```python
from build123d import *

# Parameters (mm, degrees)
F0_W     = 114.378564
F0_H     = 67.637316
F1_DEPTH = 60.96
F3_DEPTH = 12.7
F5_DEPTH = 12.7
F7_DEPTH = 86.361
F8_R     = 4.717852
F9_DEPTH = 67.638317


with BuildPart() as f1:
    # F0 (on Front) → F1 (new body)
    with BuildSketch(Plane.XZ):
        Rectangle(F0_W, F0_H)
    extrude(amount=-F1_DEPTH)

    # F2 (on face) → F3 (join)
    with BuildSketch(Plane(origin=(0, 60.96, 0), x_dir=(-1, 0, 0), z_dir=(0, 1, 0))):
        with BuildLine():
            Line((0, 33.818658), (-38.1, 33.818658))
            ThreePointArc((-38.1, 33.818658), (0, 3.86379), (38.1, 33.818658))
            Line((38.1, 33.818658), (0, 33.818658))
        make_face()
    extrude(amount=F3_DEPTH)

    # F4 (on face) → F5 (join)
    with BuildSketch(Plane.XZ):
        with BuildLine():
            ThreePointArc((-38.1, 33.818658), (0, 3.86379), (38.1, 33.818658))
            Line((38.1, 33.818658), (-38.1, 33.818658))
        make_face()
    extrude(amount=F5_DEPTH)

    # F6 (on face) → F7 (cut, through all)
    with BuildSketch(Plane.XZ.offset(12.7)):
        with BuildLine():
            Line((0, 33.818658), (-25.4, 33.818658))
            ThreePointArc((-25.4, 33.818658), (0, 19.955179), (25.4, 33.818658))
            Line((25.4, 33.818658), (0, 33.818658))
        make_face()
    extrude(amount=-F7_DEPTH, mode=Mode.SUBTRACT)

    # F8 (on face) → F9 (cut, through all)
    with BuildSketch(Plane.XY.offset(33.818658)):
        with Locations((-49.857318, 30.48)):
            Circle(F8_R)
        with Locations((49.857318, 30.48)):
            Circle(F8_R)
    extrude(amount=-F9_DEPTH, mode=Mode.SUBTRACT)


solid = f1.part
```
The model under review builds one solid part; all positions refer to its coordinate system, in mm. A direction names the side the tool comes from. Round coordinates to 2 decimals unless told otherwise and drop trailing zeros. Loops run counter-clockwise (first coordinate to the right, second up) from the corner with the lowest first, then second, coordinate; pieces in that order, holes last.
1) The part is to be moulded in two halves that separate along X. For faces 1 (the face through (57.189, 30, 0)), 2 (the face through (-1, -12.7, 19)), 3 (the face through (-53, 34, 0)), 4 (the face through (-0.42, 29.88, 19.96)), say which applies: pulls with the +X half, pulls with the -X half, needs draft (parallel to the pull), parting line crosses it, or undercut.
Values follow:
face 1: pulls with the +X half
face 2: needs draft
face 3: undercut
face 4: undercut
2) Consider section A-A on y = 30.48. State the section outline as (x, z) points.
Values follow:
outline: (-57.19, -33.82) - (-54.58, -33.82) - (-54.58, 33.82) - (-57.19, 33.82) - close; (-45.14, -33.82) - (45.14, -33.82) - (45.14, 33.82) - (25.4, 33.82) arc R30.2 cw to (-25.4, 33.82) - (-45.14, 33.82) - close; (54.58, -33.82) - (57.19, -33.82) - (57.19, 33.82) - (54.58, 33.82) - close
3) Clearance check with flat-ended pins moving along their axes: P1, Ø4, axis at x = -32, z = -9.5, coming from the -Y side; P2, Ø5, axis at x = 21.5, z = -26.5, coming from the +Y side; P3, Ø2, axis at x = -23, y = 64, coming from the -Z side; P4, Ø7.5, axis at x = -49.86, y = 30.48, coming from the +Z side. State where each tip first meets the part, or that it passes through.
Values follow:
P1: stops at y = 0
P2: stops at y = 60.96
P3: stops at z = 10.62
P4: passes through
4) Consider section D-D on y = 65. State the section outline as (x, z) points.
Values follow:
outline: (-38.1, 33.82) arc R39.21 ccw to (38.1, 33.82) - (25.4, 33.82) arc R30.2 cw to (-25.4, 33.82) - close
5) Wall thickness on line 1 along X through (y, z) = (30, 5); line 2 along X through (y, z) = (30.5, -8.5); line 3 along Y through (x, z) = (-49.5, 16): over which ranges is each line inside the solid? List them lowest first.
Values follow:
line 1: x = -57.19 to -54.55, -45.16 to 45.16, 54.55 to 57.19
line 2: x = -57.19 to -54.58, -45.14 to 45.14, 54.58 to 57.19
line 3: y = 0 to 25.78, 35.18 to 60.96
6) Consider section C-C on x = -28. State the section outline as (y, z) points.
Values follow:
outline: (-12.7, 15.63) - (0, 15.63) - (0, -33.82) - (60.96, -33.82) - (60.96, 15.63) - (73.66, 15.63) - (73.66, 33.82) - (-12.7, 33.82) - close
7) Consider section B-B on z = -24. State the section outline as (x, y) points.
Values follow:
outline: (-57.19, 0) - (57.19, 0) - (57.19, 60.96) - (-57.19, 60.96) - close; hole circle Ø9.44 at (-49.86, 30.48); hole circle Ø9.44 at (49.86, 30.48)
8) Tool access review of faces 5 (the face through (-0.73, -6.26, 3.87)), 6 (the face through (0.73, 67.22, 3.87)), 7 (the face through (46.38, 33.67, 0.47)): name each direction out of +Z, -Z, +X, -X, +Y, -Y from which nothing blocks a thin tool from reaching the whole face with its end or side.
Values follow:
face 5: -Z, -Y
face 6: -Z, +Y
face 7: +Z, -Z
